Build history of the part. All positions in model axes, mm. A direction names the side the tool comes from. Coordinates: 2 decimals unless noted, no trailing zeros. Write each loop counter-clockwise with the first axis right and the second up, starting at its lowest first coordinate (ties: lowest second). Pieces come first, ordered by that corner, then holes. Notation, with made-up numbers: (43, 20.25) -> (101, 20.25) arc R16 ccw to (101, 29.25) -> close; hole circle Ø5 at (-33.5, -18.75). An arc over 180 degrees is marked (long way). Write each question's results on one line, items separated by ' | '. Start each with the question number.
Q1. Drop flat-ended pins along their axis: pin 1 Ø1.9 at (x, y) = (25.5, 2) entering from -Z; pin 2 Ø0.6 at (y, z) = (4, -15.5) entering from -X. Give the stop position or say it passes through.
Q2. Saw through at A-A on x = 19.05. Give the cut face in (y, z), and give its area (3 significant figures).
Q3. Tool access for faces 1 (the face through (18, 3, -12.7)), 2 (the face through (127, 3, 0)), 3 (the face through (77.17, 3.13, -4.52)): list every direction of +Z, -Z, +X, -X, +Y, -Y with a clear straight run to the whole face (end or side of a thin tool).
Q4. Two-plate mould, pull along Z, no slides. Class faces 4 (the face through (33, 3, 0)), 5 (the face through (88, 6.35, -10)), 6 (the face through (11.39, 3.13, -3.85)), 7 (the face through (110, 3, -19.05)): released by +Z, released by -Z, zero draft, split by the parting line, or undercut.
Q5. Saw through at B-B on y = 1. Count the separate pieces of the cut face and the enclosed holes in it, and give its area (3 significant figures).
Q6. Drill centre lines: line 1 (X direction, y = 4.75, z = -10); line 2 (X direction, y = 5.75, z = -9.25); line 3 (X direction, y = 5.75, z = -4.5). Where is each one in solid material? Low to high.
from build123d import *

# Parameters (mm, degrees)
BOSS_EXTRUDE1_DEPTH             = 6.35
F_32_0_116_DIAMETER_HOLE1_D     = 2.9464
F_32_0_116_DIAMETER_HOLE1_DEPTH = 7.62
F_32_0_116_DIAMETER_HOLE1_TIP   = 0.885187864
F_4_40_TAPPED_HOLE1_D           = 2.2606


with BuildPart() as part:
    # Sketch1 → Boss-Extrude1 (new body)
    with BuildSketch(Plane(origin=(0, 0, 0), x_dir=(1, 0, 0), z_dir=(0, 1, 0))):
        with BuildLine():
            Line((0, 0), (67.945, 0))
            Line((67.945, 0), (69.791491908, 8.924051134))
            ThreePointArc((69.791491908, 8.924051134), (73.025, 11.557), (76.258508092, 8.924051134))
            Line((76.258508092, 8.924051134), (78.105, 0))
            Line((78.105, 0), (177.8, 0))
            Line((177.8, 0), (177.8, 19.05))
            Line((177.8, 19.05), (40.64, 19.05))
            ThreePointArc((40.64, 19.05), (38.843948776, 18.306051224), (38.1, 16.51))
            Line((38.1, 16.51), (38.1, 15.24))
            ThreePointArc((38.1, 15.24), (37.356051224, 13.443948776), (35.56, 12.7))
            Line((35.56, 12.7), (0, 12.7))
            Line((0, 12.7), (0, 0))
        make_face()
    extrude(amount=BOSS_EXTRUDE1_DEPTH)

    # #32 (0.116) Diameter Hole1
    with Locations(Plane(origin=(6.35, 6.35, -9.525), x_dir=(0, 0, 1), z_dir=(0, 1, 0))):
        with Locations((0, 0), (0, 12.7), (6.35, 6.35)):
            Hole(F_32_0_116_DIAMETER_HOLE1_D / 2, depth=F_32_0_116_DIAMETER_HOLE1_DEPTH)
            with Locations((0, 0, -(F_32_0_116_DIAMETER_HOLE1_DEPTH + F_32_0_116_DIAMETER_HOLE1_TIP / 2))):  # 118° drill point
                Cone(0, F_32_0_116_DIAMETER_HOLE1_D / 2, F_32_0_116_DIAMETER_HOLE1_TIP, mode=Mode.SUBTRACT)

    # #4-40 Tapped Hole1 (through all)
    with Locations(Plane(origin=(0, 0, -19.05), x_dir=(-1, 0, 0), z_dir=(0, 0, -1))):
        with Locations((-73.025, 3.175)):
            Hole(F_4_40_TAPPED_HOLE1_D / 2)


solid = part.part
Returned:
1) pin 1: stops at z = -12.7 | pin 2: stops at x = 38.1
2) outline: (0, -12.7) -> (6.35, -12.7) -> (6.35, -11) -> (0, -11) -> close; (0, -8.05) -> (6.35, -8.05) -> (6.35, 0) -> (0, 0) -> close | area: 61.9 mm2
3) face 1: -Z, -X, +Y, -Y | face 2: +Z, +X, -X, +Y, -Y | face 3: +Z, +Y, -Y
4) face 4: released by +Z | face 5: zero draft | face 6: undercut | face 7: released by -Z
5) separate pieces: 1 | enclosed holes: 3 | area: 3,040 mm2
6) line 1: x = 0 to 4.96, 7.74 to 17.66, 20.44 to 70.22, 75.83 to 177.8 | line 2: x = 0 to 4.9, 7.8 to 17.6, 20.5 to 69.88, 76.17 to 177.8 | line 3: x = 0 to 12.06, 13.34 to 68.88, 77.17 to 177.8
